Check sheet for the modelled part. Datum: model origin and axes. Units: mm. A direction names the side the tool comes from. Round coordinates to 2 decimals unless told otherwise and drop trailing zeros. Order: outer loops, then holes, each group sorted by start corner. A loop starts at its lowest first (then second) coordinate and runs counter-clockwise, first axis right, second up. Notation, with made-up numbers: M 56.25,-14.5 L 79.25,-14.5 A21 ccw 79.25,12.5 Z; hole C -22,31.5 d3. An arc over 180 degrees is marked long. One line per item, written item: value. Start each with the question number.
(1) Cross-section at C-C, the plane y = 2. Enter the section's corners in (x, z) (3 decimals), and give its area (3 significant figures).
(2) Release check for a two-part mould opening along X. For faces 4 (the face through (-31.24, 9.86, -6.94)), 5 (the face through (8, 20, -6)), 6 (the face through (-13.064, 15.507, 7.352)), 7 (the face through (0, 17, -9.5)) record: released by +X, released by -X, zero draft, split by the parting line, or undercut.
(3) Thickness scan on L1, parallel to X at y = 8, z = 0; L2, parallel to X at y = 11.5, z = -12.5; L3, parallel to Z at x = 1, y = 1.5. Record the ranges inside material, lowest first.
(4) Depth check by flat-ended pin: pin 1 Ø6 at (x, y) = (-13.5, 3.5) entering from -Z; pin 2 Ø1.5 at (x, y) = (10, 5.5) entering from -Z; pin 3 Ø1.8 at (x, y) = (-2.5, 17) entering from +Z; pin 4 Ø5.5 at (x, z) = (2, -0.5) entering from +Y. Enter the tip coordinate at first touch or a pass-through.
(5) Cross-section at B-B, the plane z = -12.5. Enter the section's corners in (x, y).
(6) Cross-section at A-A, the plane x = 0. Enter the section's corners in (y, z) (3 decimals), and give its area (3 significant figures).
(7) Access from +Z, -Z, +X, -X, +Y, -Y to the whole of each face (thin tool, end or side, straight path). Record for faces 1 (the face through (12.9, 15.51, 7.64)), 2 (the face through (5.261, 1.479, 16.706)), 3 (the face through (-14, 0, 14)).
from build123d import *

# Parameters (mm, degrees)
SKETCH2_R                = 32
BOSS_EXTRUDE1_DEPTH      = 20
SKETCH3_R                = 10.725
CUT_EXTRUDE1_DEPTH       = 6.97
SKETCH4_R                = 13.765
CUT_EXTRUDE2_DEPTH       = 10.04
FILLET1_R                = 2
CIRPATTERN1_COUNT        = 3
FILLET1_OF_CIRPATTERN1_R = 2
SKETCH5_R                = 6.5
CUT_EXTRUDE3_DEPTH       = 20
SKETCH6_R                = 17.515
CUT_EXTRUDE4_DEPTH       = 3
SKETCH7_R                = 2.515
CUT_EXTRUDE5_DEPTH       = 20
CUT_EXTRUDE6_DEPTH       = 6


with BuildPart() as part:
    # Sketch2 → Boss-Extrude1 (new body)
    with BuildSketch(Plane(origin=(0, 0, 0), x_dir=(1, 0, 0), z_dir=(0, 1, 0))):
        with Locations(Location((0, 0, 0), (0, 0, 270))):
            Circle(SKETCH2_R)
    extrude(amount=BOSS_EXTRUDE1_DEPTH)

    # Sketch3 → Cut-Extrude1 (cut)
    with BuildSketch(Plane(origin=(0, 0, -32), x_dir=(-1, 0, 0), z_dir=(0, 0, -1))):
        with Locations((0, 20)):
            Circle(SKETCH3_R)
    cut_extrude1 = extrude(amount=-CUT_EXTRUDE1_DEPTH, mode=Mode.SUBTRACT)

    # Sketch4 → Cut-Extrude2 (cut)
    with BuildSketch(Plane(origin=(0, 0, -25.03), x_dir=(-1, 0, 0), z_dir=(0, 0, -1))):
        with Locations((0, 20)):
            Circle(SKETCH4_R)
    cut_extrude2 = extrude(amount=-CUT_EXTRUDE2_DEPTH, mode=Mode.SUBTRACT)

    # Fillet1
    fillet1_edges = [part.edges().sort_by_distance(p)[0] for p in [
        (0, 6.235, -25.03),
        (0, 6.235, -14.99),
    ]]
    fillet(fillet1_edges, radius=FILLET1_R)

    # CirPattern1: Cut-Extrude1, Cut-Extrude2 ×3 about axis
    cirpattern1_axis = Axis((0, 0, 0), (0, 1, 0))
    add([cut_extrude1.rotate(cirpattern1_axis, i * 360 / CIRPATTERN1_COUNT) for i in range(1, CIRPATTERN1_COUNT)], mode=Mode.SUBTRACT)
    add([cut_extrude2.rotate(cirpattern1_axis, i * 360 / CIRPATTERN1_COUNT) for i in range(1, CIRPATTERN1_COUNT)], mode=Mode.SUBTRACT)

    # Fillet1 of CirPattern1
    fillet1_of_cirpattern1_edges = [part.edges().sort_by_distance(p)[0] for p in [
        (-21.676615857, 6.235, 12.515),
        (-12.981720803, 6.235, 7.495),
        (21.676615857, 6.235, 12.515),
        (12.981720803, 6.235, 7.495),
    ]]
    fillet(fillet1_of_cirpattern1_edges, radius=FILLET1_OF_CIRPATTERN1_R)

    # Sketch5 → Cut-Extrude3 (cut)
    with BuildSketch(Plane(origin=(0, 20, 0), x_dir=(1, 0, 0), z_dir=(0, 1, 0))):
        with Locations(Location((0, 0, 0), (0, 0, 270))):
            Circle(SKETCH5_R)
    extrude(amount=-CUT_EXTRUDE3_DEPTH, mode=Mode.SUBTRACT)

    # Sketch6 → Cut-Extrude4 (cut)
    with BuildSketch(Plane(origin=(0, 0, 0), x_dir=(1, 0, 0), z_dir=(0, 1, 0))):
        with Locations(Location((0, 0, 0), (0, 0, 270))):
            Circle(SKETCH6_R)
    extrude(amount=CUT_EXTRUDE4_DEPTH, mode=Mode.SUBTRACT)

    # Sketch7 → Cut-Extrude5 (cut)
    with BuildSketch(Plane(origin=(0, 0, 0), x_dir=(1, 0, 0), z_dir=(0, 1, 0))):
        with Locations(Location((0, -25, 0), (0, 0, 90))):
            Circle(SKETCH7_R)
        with Locations(Location((-21.650635095, 12.5, 0), (0, 0, 90))):
            Circle(SKETCH7_R)
        with Locations(Location((21.650635095, 12.5, 0), (0, 0, 90))):
            Circle(SKETCH7_R)
    extrude(amount=CUT_EXTRUDE5_DEPTH, mode=Mode.SUBTRACT)

    # Sketch8 → Cut-Extrude6 (cut)
    with BuildSketch(Plane(origin=(0, 20, 0), x_dir=(1, 0, 0), z_dir=(0, 1, 0))):
        Polygon((5.484827557, 9.5), (-5.484827557, 9.5), (-10.969655115, 0), (-5.484827557, -9.5), (5.484827557, -9.5), (10.969655115, 0), align=None)
    extrude(amount=-CUT_EXTRUDE6_DEPTH, mode=Mode.SUBTRACT)


solid = part.part
Values found:
1. outline: C 0,0 d64; hole C -21.651,-12.5 d5.03; hole C 0,0 d35.03; hole C 0,25 d5.03; hole C 21.651,-12.5 d5.03
1. area: 2,190 mm^2
2. face 4: split by the parting line
2. face 5: zero draft
2. face 6: undercut
2. face 7: undercut
3. L1: -32 to -6.5, 6.5 to 32
3. L2: -29.46 to -24.17, -19.14 to 19.14, 24.17 to 29.46
3. L3: -31.98 to -17.49, 17.49 to 22.69, 27.31 to 31.98
4. pin 1: z = -30.23
4. pin 2: z = -30.63
4. pin 3: z = 31.96
4. pin 4: through
5. outline: M -29.46,0 L -24.17,0 L -24.17,20 L -29.46,20 Z; M -19.14,0 L -12.27,0 L -12.27,3 L 12.27,3 L 12.27,0 L 19.14,0 L 19.14,20 L -19.14,20 Z; M 24.17,0 L 29.46,0 L 29.46,20 L 24.17,20 Z
6. outline: M 0,-32 L 9.275,-32 L 9.275,-25.03 L 8.235,-25.03 A2 cw 6.235,-23.03 L 6.235,-16.99 A2 cw 8.235,-14.99 L 20,-14.99 L 20,-9.5 L 14,-9.5 L 14,-6.5 L 3,-6.5 L 3,-17.515 L 0,-17.515 Z; M 0,17.515 L 3,17.515 L 3,6.5 L 14,6.5 L 14,9.5 L 20,9.5 L 20,22.485 L 0,22.485 Z; M 0,27.515 L 20,27.515 L 20,32 L 0,32 Z
6. area: 606 mm^2
7. face 1: +Y
7. face 2: -Y
7. face 3: +Z, -Z, +X, -X, -Y
